from build123d import *

# Parameters (mm, degrees)
CROQUIS1_R              = 10
SALIENTE_EXTRUIR1_DEPTH = 1
CROQUIS2_R              = 3.5
SALIENTE_EXTRUIR2_DEPTH = 10
CROQUIS3_R              = 3
CORTAR_EXTRUIR1_DEPTH   = 10
CORTAR_EXTRUIR2_DEPTH   = 10


with BuildPart() as part:
    # Croquis1 → Saliente-Extruir1 (new body)
    with BuildSketch(Plane.XY):
        Circle(CROQUIS1_R)
    extrude(amount=SALIENTE_EXTRUIR1_DEPTH)

    # Croquis2 → Saliente-Extruir2 (add)
    with BuildSketch(Plane.XY.offset(1)):
        Circle(CROQUIS2_R)
    extrude(amount=SALIENTE_EXTRUIR2_DEPTH)

    # Croquis3 → Cortar-Extruir1 (cut)
    with BuildSketch(Plane.XY.offset(11)):
        Circle(CROQUIS3_R)
    extrude(amount=-CORTAR_EXTRUIR1_DEPTH, mode=Mode.SUBTRACT)

    # Croquis4 → Cortar-Extruir2 (cut)
    with BuildSketch(Plane(origin=(0, 0, 0), x_dir=(1, 0, 0), z_dir=(0, 1, 0))):
        with BuildLine():
            ThreePointArc((1.25, -5.834936491), (0, -5.5), (-1.25, -5.834936491))
            ThreePointArc((-1.25, -5.834936491), (-1.833451245, -6.300454022), (-2.253469547, -6.917468245))
            ThreePointArc((-2.253469547, -6.917468245), (-2.5, -8), (-2.253469547, -9.082531755))
            ThreePointArc((-2.253469547, -9.082531755), (-1.833451245, -9.699545978), (-1.25, -10.165063509))
            ThreePointArc((-1.25, -10.165063509), (0, -10.5), (1.25, -10.165063509))
            ThreePointArc((1.25, -10.165063509), (1.833451245, -9.699545978), (2.253469547, -9.082531755))
            ThreePointArc((2.253469547, -9.082531755), (2.5, -8), (2.253469547, -6.917468245))
            ThreePointArc((2.253469547, -6.917468245), (1.833451245, -6.300454022), (1.25, -5.834936491))
        make_face()
    cortar_extruir2 = extrude(amount=-CORTAR_EXTRUIR2_DEPTH, mode=Mode.SUBTRACT)

    # Simetría1: Cortar-Extruir2 across plane
    add(cortar_extruir2.mirror(Plane.ZX), mode=Mode.SUBTRACT)


solid = part.part
Can you work these out from the model? Positions are in its coordinate system, mm. A direction names the side the tool comes from. Coordinates: 2 decimals unless noted, no trailing zeros. Write each loop counter-clockwise with the first axis right and the second up, starting at its lowest first coordinate (ties: lowest second). Pieces come first, ordered by that corner, then holes. Notation, with made-up numbers: (56.25, 54.5) - (74.25, 54.5) arc R22 ccw to (74.25, 84.5) - close; hole circle Ø7 at (75.5, -28). An arc over 180 degrees is marked (long way). Return JSON: item names as keys, results as strings. Group by question number.
Item 1: If we section it at C-C (y = -0.5): Write out the boundary of the cut face in (x, z).
Item 2: I'm going to push flat-ended pins straight in: pin 1 Ø4 at (y, z) = (-6, 9.5) entering from -X; pin 2 Ø1 at (x, z) = (1.5, 3) entering from +Y; pin 3 Ø3.5 at (x, y) = (0, 0) entering from +Z; pin 4 Ø5 at (y, z) = (5, 1.5) entering from +X. Where does each tip first touch, or does it pass through?
Item 3: If we section it at B-B (x = 0): Write out the boundary of the cut face in (y, z), then the cut area to 3 significant figures.
Item 4: If we section it at D-D (z = 1.25): Write out the boundary of the cut face in (x, y).
Item 5: If we section it at A-A (z = 6.5): Write out the boundary of the cut face in (x, y), then the cut area to 3 significant figures.
Item 6: Which directions (+Z, -Z, +X, -X, +Y, -Y) give clear straight access to the entire face, cutting with the end or side of a thin tool? Please do faces 4 (the face through (-2.17, -9.76, 0.49)), 5 (the face through (0, -4, 1)).
Item 7: Please list where these lines run through material, in increasing order: probe 1 along Y at (x, z) = (0, 4.75); probe 2 along Z at (x, y) = (-4.75, -2.75); probe 3 along X at (y, z) = (-0.5, 7.5).
Item 8: We'd pull the mould along Y, two halves only. Please class faces 1 (the face through (2.86, 0.9, 6.07)), 2 (the face through (3, 1, 11)), 3 (the face through (-3.497, 0.154, 5.93)): pulls with the +Y half, pulls with the -Y half, needs draft (parallel to the pull), parting line crosses it, or undercut.
Return value:
{
 "1": {"outline": "(-9.99, 0) - (9.99, 0) - (9.99, 1) - (3.46, 1) - (3.46, 11) - (2.96, 11) - (2.96, 1) - (-2.96, 1) - (-2.96, 11) - (-3.46, 11) - (-3.46, 1) - (-9.99, 1) - close"},
 "2": {"pin 1": "passes through", "pin 2": "stops at y = 3.35", "pin 3": "stops at z = 1", "pin 4": "stops at x = 9.67"},
 "3": {"outline": "(-10, 0) - (10, 0) - (10, 1) - (3.5, 1) - (3.5, 5.5) - (3, 5.5) - (3, 1) - (-3, 1) - (-3, 5.5) - (-3.5, 5.5) - (-3.5, 1) - (-10, 1) - close; (-3.5, 10.5) - (-3, 10.5) - (-3, 11) - (-3.5, 11) - close; (3, 10.5) - (3.5, 10.5) - (3.5, 11) - (3, 11) - close", "area": "25.0 mm^2"},
 "4": {"outline": "circle Ø7 at (0, 0); hole circle Ø6 at (0, 0)"},
 "5": {"outline": "(-2, -2.87) - (-2, -2.24) arc R3 cw to (-2, 2.24) - (-2, 2.87) arc R3.5 ccw to start; (2, -2.87) arc R3.5 ccw to (2, 2.87) - (2, 2.24) arc R3 cw to (2, -2.24) - close", "area": "5.90 mm^2"},
 "6": {"face 4": "+Z, -Z", "face 5": "+Z"},
 "7": {"probe 1": "y = -3.5 to -3, 3 to 3.5", "probe 2": "z = 0 to 1", "probe 3": "x = -3.46 to -2.96, 2.96 to 3.46"},
 "8": {"face 1": "undercut", "face 2": "needs draft", "face 3": "parting line crosses it"}
}
